Could you check a few things on this model? Use its own coordinates, in mm. A direction names the side the tool comes from. Give positions to 0.01 mm unless a question says otherwise; leave off trailing zeros. Order: outer loops, then holes, each group sorted by start corner. A loop starts at its lowest first (then second) coordinate and runs counter-clockwise, first axis right, second up.
(1) Will these pins go through, and if not, where does the flat tip stop? pin 1 (9 mm diameter, centred on x = 13.6, y = 32.5, fed in from -Z); pin 2 (5 mm diameter, centred on x = 128, y = 32.5, fed in from +Z).
(2) Imagine slicing it at D-D, the plane x = 13.6. Write out the boundary of the cut face in (y, z).
(3) On a 3-axis mill with a long thin cutter (end or side, diameter ignored), from which of +Z, -Z, +X, -X, +Y, -Y can I reach the whole of each face in a straight line? I mean faces 4 (the flat face through (124, 30, 6.4)), 5 (the flat face through (69, 65, 5)), 6 (the cylindrical face through (18.37, 34, 9.51)), 7 (the cylindrical face through (111.844, 6.407, 4.93)). Say none if no direction works.
(4) Imagine slicing it at A-A, the plane x = 61. Write out the boundary of the cut face in (y, z).
(5) If we mould it in two halves opening along X, with no side actions, what happens to faces 1 (the flat face through (69, 0, 5)), 2 (the flat face through (0, 32, 5)), 3 (the cylindrical face through (28.156, 6.407, 4.93))? For each: released by +X, released by -X, zero draft, split by the parting line, or undercut.
(6) Imagine slicing it at C-C, the plane z = 4. Write out the boundary of the cut face in (x, y), then the cut area to 3 significant figures.
(7) If I drill on probe 1 along X at (y, z) = (22, 9.75); probe 2 along Y at (x, z) = (31, 7.75); probe 3 along Y at (x, z) = (13.6, 3.75), over which ranges is the centre line in solid material (lowest first)?
(8) Imagine slicing it at B-B, the plane y = 32.5. State how many separate pieces and enclosed holes the cut face has, then the cut area to 3 significant figures.
from build123d import *

# Parameters (mm, degrees)
SKETCH_1_W                   = 140
SKETCH_1_H                   = 65
EXTRUDE_1_DEPTH              = 10
SKETCH_2_W                   = 85.6
SKETCH_2_H                   = 54
CUT_EXTRUDE_1_DEPTH          = 11
FILLET_1_R                   = 3.18
HOLE_WIZARD_M6_1_D           = 6.6
HOLE_WIZARD_M6_1_DEPTH       = 15
HOLE_WIZARD_M6_1_CBORE_D     = 11
HOLE_WIZARD_M6_1_CBORE_DEPTH = 6.4
HOLE_WIZARD_M6_1_TIP         = 1.982840043
SKETCH_6_R                   = 5
CUT_EXTRUDE_3_DEPTH          = 1


with BuildPart() as part:
    # 草图1 → 凸台-拉伸1 (new body)
    with BuildSketch(Plane.XY):
        with Locations((70, 32.5)):
            Rectangle(SKETCH_1_W, SKETCH_1_H)
    extrude(amount=EXTRUDE_1_DEPTH)

    # 草图2 → 切除-拉伸1 (cut, through all)
    with BuildSketch(Plane.XY.offset(10)):
        with Locations((70, 32.5)):
            Rectangle(SKETCH_2_W, SKETCH_2_H)
    extrude(amount=-CUT_EXTRUDE_1_DEPTH, mode=Mode.SUBTRACT)

    # 圆角1
    fillet_1_edges = [part.edges().sort_by_distance(p)[0] for p in [
        (27.2, 5.5, 5),
        (27.2, 59.5, 5),
        (112.8, 59.5, 5),
        (112.8, 5.5, 5),
    ]]
    fillet(fillet_1_edges, radius=FILLET_1_R)

    # M6 六角凹头螺钉的柱形沉头孔1
    with Locations(Plane(origin=(0, 0, 0), x_dir=(-1, 0, 0), z_dir=(0, 0, -1))):
        with Locations((-126.4, 32.5), (-13.6, 32.5)):
            CounterBoreHole(HOLE_WIZARD_M6_1_D / 2, HOLE_WIZARD_M6_1_CBORE_D / 2, HOLE_WIZARD_M6_1_CBORE_DEPTH, depth=HOLE_WIZARD_M6_1_DEPTH)
            with Locations((0, 0, -(HOLE_WIZARD_M6_1_DEPTH + HOLE_WIZARD_M6_1_TIP / 2))):  # 118° drill point
                Cone(0, HOLE_WIZARD_M6_1_D / 2, HOLE_WIZARD_M6_1_TIP, mode=Mode.SUBTRACT)

    # 草图6 → 切除-拉伸3 (cut)
    with BuildSketch(Plane.XY.offset(10)):
        with Locations((13.6, 32.5)):
            Circle(SKETCH_6_R)
        with Locations((126.4, 32.5)):
            Circle(SKETCH_6_R)
    extrude(amount=-CUT_EXTRUDE_3_DEPTH, mode=Mode.SUBTRACT)


solid = part.part
Answer block:
1. pin 1: stops at z = 6.4
1. pin 2: stops at z = 9
2. outline: (0, 0) - (27, 0) - (27, 6.4) - (29.2, 6.4) - (29.2, 9) - (27.5, 9) - (27.5, 10) - (0, 10) - close; (35.8, 6.4) - (38, 6.4) - (38, 0) - (65, 0) - (65, 10) - (37.5, 10) - (37.5, 9) - (35.8, 9) - close
3. face 4: -Z
3. face 5: +Z, -Z, +X, -X, +Y
3. face 6: +Z
3. face 7: +Z, -Z
4. outline: (0, 0) - (5.5, 0) - (5.5, 10) - (0, 10) - close; (59.5, 0) - (65, 0) - (65, 10) - (59.5, 10) - close
5. face 1: zero draft
5. face 2: released by -X
5. face 3: undercut
6. outline: (0, 0) - (140, 0) - (140, 65) - (0, 65) - close; hole circle Ø11 at (13.6, 32.5); hole (27.2, 8.68) arc R3.18 ccw to (30.38, 5.5) - (109.62, 5.5) arc R3.18 ccw to (112.8, 8.68) - (112.8, 56.32) arc R3.18 ccw to (109.62, 59.5) - (30.38, 59.5) arc R3.18 ccw to (27.2, 56.32) - close; hole circle Ø11 at (126.4, 32.5)
6. area: 4,300 mm2
7. probe 1: x = 0 to 27.2, 112.8 to 140
7. probe 2: y = 0 to 5.5, 59.5 to 65
7. probe 3: y = 0 to 27, 38 to 65
8. separate pieces: 4
8. enclosed holes: 0
8. area: 349 mm2
